Can you work these out from the model? Positions are in its coordinate system, mm. Face numbers are marked on the shaded views. A direction names the side the tool comes from. Give positions to 0.01 mm unless a question says otherwise; leave off trailing zeros. Loops run counter-clockwise (first coordinate to the right, second up) from the corner with the lowest first, then second, coordinate; pieces in that order, holes last. Notation, with made-up numbers: (16.25, 73.5) -> (75.25, 73.5) arc R22 cw to (75.25, 112.5) -> close; hole circle Ø10 at (-39, 11.25). An arc over 180 degrees is marked (long way). Return JSON: item names as keys, results as strings. Group by question number.
Q1. Which directions (+Z, -Z, +X, -X, +Y, -Y) give clear straight access to the entire face, cutting with the end or side of a thin tool? Please do the marked faces 1, 2 and 3.
Q2. Suppose I cut it at B-B, the plane x = 190. Please give me the cut outline in (y, z), and give its area (3 significant figures).
Q3. Suppose I cut it at A-A, the plane z = 15. Count the separate pieces of the cut face and the enclosed holes in it, and give its area (3 significant figures).
Q4. I need wall thicknesses on line 1 along Z through (x, y) = (190, 32); line 2 along X through (y, z) = (36, 13); line 3 along X through (y, z) = (26, 21). Which ranges of each line are inside material? Lowest first, please. Write a range as [from, to].
Q5. Suppose I cut it at D-D, the plane x = 137. Please give me the cut outline in (y, z), and give its area (3 significant figures).
Q6. Suppose I cut it at C-C, the plane z = 42.5. Please give me the cut outline in (x, y).
Q7. Will these pins go through, and if not, where does the flat tip stop? pin 1 (7.5 mm diameter, centred on y = -19, z = 3, fed in from -X); pin 2 (12 mm diameter, centred on x = 215.5, z = -37.5, fed in from +Y); pin 3 (3 mm diameter, centred on y = 6.5, z = 5, fed in from +X); pin 4 (4.5 mm diameter, centred on y = 100.5, z = -31.5, fed in from +X).
Q8. Thinking about a two-plate mould opening in X: for the marked faces 4, 5, 6 and 7, which applies, pulls with the +X half, pulls with the -X half, needs draft (parallel to the pull), parting line crosses it, or undercut?
```python
from build123d import *

# Parameters (mm, degrees)
BOSS_EXTRUDE1_DEPTH = 50
CUT_EXTRUDE1_DEPTH  = 268.675176286
CUT_EXTRUDE3_DEPTH  = 35
SKETCH6_W           = 70
SKETCH6_H           = 70
CUT_EXTRUDE4_DEPTH  = 55
SKETCH7_R           = 22.5
CUT_EXTRUDE5_DEPTH  = 246.662369931
FILLET1_R           = 25
FILLET2_R           = 5
FILLET3_R           = 5


with BuildPart() as part:
    # Sketch1 → Boss-Extrude1 (new, symmetric)
    with BuildSketch(Plane.XY):
        with BuildLine():
            Line((0, 0), (40, 0))
            Line((40, 0), (40, -35))
            Line((40, -35), (155, -35))
            Line((155, -35), (155, 10))
            Line((155, 10), (225, 10))
            Line((225, 10), (225, 85))
            Line((225, 85), (205, 85))
            Line((205, 85), (205, 105))
            Line((205, 105), (105, 105))
            ThreePointArc((105, 105), (68.0448187, 97.649157401), (36.715728753, 76.715728753))
            Line((36.715728753, 76.715728753), (0, 40))
            Line((0, 40), (0, 0))
        make_face()
    extrude(amount=BOSS_EXTRUDE1_DEPTH, both=True)

    # Sketch2 → Cut-Extrude1 (cut, through all)
    with BuildSketch(Plane.XY.offset(50)):
        with BuildLine():
            Line((40, 58.786796564), (40, 20))
            Line((40, 20), (122, 20))
            Line((122, 20), (122, 90))
            Line((122, 90), (105, 90))
            ThreePointArc((105, 90), (73.785070185, 83.790964413), (47.32233047, 66.109127035))
            Line((47.32233047, 66.109127035), (40, 58.786796564))
        make_face()
    extrude(amount=-CUT_EXTRUDE1_DEPTH, mode=Mode.SUBTRACT)

    # Sketch5 → Cut-Extrude3 (cut, symmetric)
    with BuildSketch(Plane.XY):
        with BuildLine():
            Line((205, 95), (105, 95))
            ThreePointArc((105, 95), (71.871653023, 88.410362075), (43.786796564, 69.644660941))
            Line((43.786796564, 69.644660941), (0, 25.857864376))
            Line((0, 25.857864376), (0, 40))
            Line((0, 40), (36.715728753, 76.715728753))
            ThreePointArc((36.715728753, 76.715728753), (68.0448187, 97.649157401), (105, 105))
            Line((105, 105), (205, 105))
            Line((205, 105), (205, 95))
        make_face()
    extrude(amount=CUT_EXTRUDE3_DEPTH, both=True, mode=Mode.SUBTRACT)

    # Sketch6 → Cut-Extrude4 (cut)
    with BuildSketch(Plane(origin=(0, 105, 0), x_dir=(1, 0, 0), z_dir=(0, 1, 0))):
        with Locations((190, -15)):
            Rectangle(SKETCH6_W, SKETCH6_H)
    extrude(amount=-CUT_EXTRUDE4_DEPTH, mode=Mode.SUBTRACT)

    # Sketch7 → Cut-Extrude5 (cut, through all)
    with BuildSketch(Plane(origin=(0, 50, 0), x_dir=(1, 0, 0), z_dir=(0, 1, 0))):
        with Locations(Location((190, -15, 0), (0, 0, 180))):
            Circle(SKETCH7_R)
    extrude(amount=-CUT_EXTRUDE5_DEPTH, mode=Mode.SUBTRACT)

    # Fillet1
    fillet1_edges = [part.edges().sort_by_distance(p)[0] for p in [
        (225, 30, 50),
    ]]
    fillet(fillet1_edges, radius=FILLET1_R)

    # Fillet2
    fillet2_edges = [part.edges().sort_by_distance(p)[0] for p in [
        (155, 10, 0),
        (155, -35, 0),
        (40, -35, 0),
        (40, 0, 0),
        (0, 0, 0),
        (205, 85, -35),
    ]]
    fillet(fillet2_edges, radius=FILLET2_R)

    # Fillet3
    fillet3_edges = [part.edges().sort_by_distance(p)[0] for p in [
        (122, 90, 0),
        (122, 20, 0),
        (40, 20, 0),
        (40, 58.786796564, 0),
    ]]
    fillet(fillet3_edges, radius=FILLET3_R)


solid = part.part
```
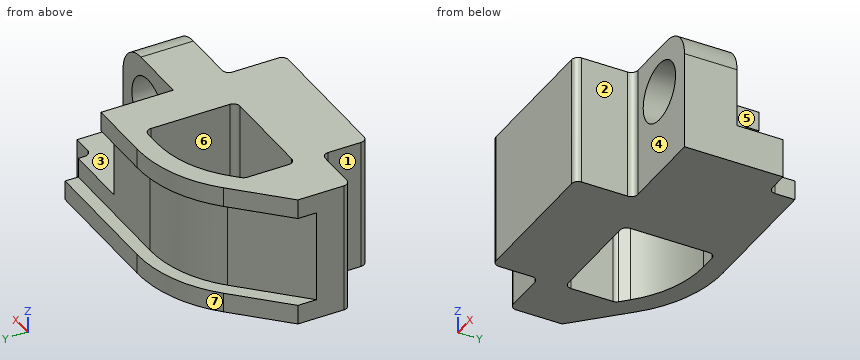
Ans:
{
 "1": {"face 1": "+Z, -Z, -X, -Y", "face 2": "+Z, -Z, +X, -Y", "face 3": "+Z, +X, +Y"},
 "2": {"outline": "(10, -50) -> (105, -50) -> (105, -35) -> (95, -35) -> (95, -20) -> (50, -20) -> (50, -7.5) -> (10, -7.5) -> close; (10, 37.5) -> (50, 37.5) -> (50, 50) -> (10, 50) -> close", "area": "3,700 mm^2"},
 "3": {"separate pieces": "2", "enclosed holes": "1", "area": "12,100 mm^2"},
 "4": {"line 1": "z = [-50, -7.5], [37.5, 50]", "line 2": "x = [10.14, 40], [122, 167.59], [212.41, 225]", "line 3": "x = [0.14, 40], [122, 168.31], [211.69, 225]"},
 "5": {"outline": "(-35, -50) -> (105, -50) -> (105, -35) -> (95, -35) -> (95, 35) -> (105, 35) -> (105, 50) -> (-35, 50) -> close", "area": "13,300 mm^2"},
 "6": {"outline": "(0, 5) arc R5 ccw to (5, 0) -> (35, 0) arc R5 cw to (40, -5) -> (40, -30) arc R5 ccw to (45, -35) -> (150, -35) arc R5 ccw to (155, -30) -> (155, 5) arc R5 cw to (160, 10) -> (217.85, 10) -> (217.85, 50) -> (155, 50) -> (155, 105) -> (105, 105) arc R96.57 ccw to (36.72, 76.72) -> (0, 40) -> close; hole (40, 25) arc R5 ccw to (45, 20) -> (117, 20) arc R5 ccw to (122, 25) -> (122, 85) arc R5 ccw to (117, 90) -> (105, 90) arc R81.57 ccw to (47.32, 66.11) -> (41.46, 60.25) arc R5 ccw to (40, 56.72) -> close"},
 "7": {"pin 1": "stops at x = 40", "pin 2": "stops at y = 85.03", "pin 3": "stops at x = 156", "pin 4": "passes through"},
 "8": {"face 4": "needs draft", "face 5": "pulls with the +X half", "face 6": "undercut", "face 7": "pulls with the -X half"}
}
